from build123d import *

# Parameters (mm, degrees)
SKETCH1_W           = 13.2
SKETCH1_H           = 12.7
BOSS_EXTRUDE1_DEPTH = 9.5
SKETCH2_R           = 3
BOSS_EXTRUDE2_DEPTH = 8.8
SKETCH4_R           = 2.5
CUT_EXTRUDE1_DEPTH  = 2
SKETCH5_R           = 1.5
BOSS_EXTRUDE3_DEPTH = 13
REVOLVE2_ANGLE      = 180
FILLET1_R           = 1
SKETCH6_W           = 0.8
SKETCH6_H           = 2
BOSS_EXTRUDE4_DEPTH = 4
SKETCH7_W           = 1
SKETCH7_H           = 2
CUT_EXTRUDE2_DEPTH  = 33.182332109
FILLET2_R           = 0.5


with BuildPart() as part:
    # Sketch1 → Boss-Extrude1 (new body)
    with BuildSketch(Plane(origin=(0, 0, 0), x_dir=(1, 0, 0), z_dir=(0, 1, 0))):
        Rectangle(SKETCH1_W, SKETCH1_H)
    extrude(amount=BOSS_EXTRUDE1_DEPTH)

    # Sketch2 → Boss-Extrude2 (add)
    with BuildSketch(Plane(origin=(0, 9.5, 0), x_dir=(1, 0, 0), z_dir=(0, 1, 0))):
        with Locations(Location((0, 0, 0), (0, 0, 270))):
            Circle(SKETCH2_R)
    extrude(amount=BOSS_EXTRUDE2_DEPTH)

    # Sketch4 → Cut-Extrude1 (cut)
    with BuildSketch(Plane(origin=(0, 18.3, 0), x_dir=(1, 0, 0), z_dir=(0, 1, 0))):
        with Locations(Location((0, 0, 0), (0, 0, 270))):
            Circle(SKETCH4_R)
    extrude(amount=-CUT_EXTRUDE1_DEPTH, mode=Mode.SUBTRACT)

    # Sketch5 → Boss-Extrude3 (add)
    with BuildSketch(Plane(origin=(0, 16.3, 0), x_dir=(1, 0, 0), z_dir=(0, 1, 0))):
        with Locations(Location((0, 0, 0), (0, 0, 90))):
            Circle(SKETCH5_R)
    extrude(amount=BOSS_EXTRUDE3_DEPTH)

    # Sketch3 → Revolve2 (revolve)
    with BuildSketch(Plane(origin=(0, 16.3, 0), x_dir=(1, 0, 0), z_dir=(0, 1, 0))):
        with BuildLine():
            Line((0, -2.5), (0, 2.5))
            ThreePointArc((0, 2.5), (-2.5, 0), (0, -2.5))
        make_face()
    revolve(axis=Axis((0, 16.3, 3), (0, 0, -1)), revolution_arc=REVOLVE2_ANGLE)

    # Fillet1
    fillet1_edges = [part.edges().sort_by_distance(p)[0] for p in [
        (0, 29.3, 1.5),
    ]]
    fillet(fillet1_edges, radius=FILLET1_R)

    # Sketch6 → Boss-Extrude4 (add)
    with BuildSketch(Plane.XZ):
        with Locations((-4.7, 2.4)):
            Rectangle(SKETCH6_W, SKETCH6_H)
        with Locations((-4.7, -2.4)):
            Rectangle(SKETCH6_W, SKETCH6_H)
        with Locations((0, -2.4)):
            Rectangle(SKETCH6_W, SKETCH6_H)
        with Locations((0, 2.4)):
            Rectangle(SKETCH6_W, SKETCH6_H)
        with Locations((4.7, 2.4)):
            Rectangle(SKETCH6_W, SKETCH6_H)
        with Locations((4.7, -2.4)):
            Rectangle(SKETCH6_W, SKETCH6_H)
    extrude(amount=BOSS_EXTRUDE4_DEPTH)

    # Sketch7 → Cut-Extrude2 (cut, through all)
    with BuildSketch(Plane.ZY.offset(5.1)):
        with Locations((-2.4, -2.5)):
            Rectangle(SKETCH7_W, SKETCH7_H)
        with Locations((2.4, -2.5)):
            Rectangle(SKETCH7_W, SKETCH7_H)
    extrude(amount=-CUT_EXTRUDE2_DEPTH, mode=Mode.SUBTRACT)

    # Fillet2
    fillet2_edges = [part.edges().sort_by_distance(p)[0] for p in [
        (4.7, -3.5, 2.9),
        (4.7, -3.5, 1.9),
        (4.7, -3.5, -1.9),
        (4.7, -3.5, -2.9),
        (4.7, -1.5, -1.9),
        (4.7, -1.5, 2.9),
        (4.7, -1.5, 1.9),
        (4.7, -1.5, -2.9),
        (0, -1.5, 1.9),
        (0, -1.5, 2.9),
        (0, -3.5, 2.9),
        (0, -3.5, 1.9),
        (0, -3.5, -1.9),
        (0, -3.5, -2.9),
        (0, -1.5, -2.9),
        (0, -1.5, -1.9),
        (-4.7, -3.5, 2.9),
        (-4.7, -1.5, 2.9),
        (-4.7, -3.5, 1.9),
        (-4.7, -1.5, 1.9),
        (-4.7, -1.5, -1.9),
        (-4.7, -1.5, -2.9),
        (-4.7, -3.5, -1.9),
        (-4.7, -3.5, -2.9),
        (0, -4, -1.4),
        (0, -4, -3.4),
        (4.7, -4, -1.4),
        (4.7, -4, -3.4),
        (4.7, -4, 1.4),
        (4.7, -4, 3.4),
        (0, -4, 3.4),
        (0, -4, 1.4),
        (-4.7, -4, 3.4),
        (-4.7, -4, 1.4),
        (-4.7, -4, -1.4),
        (-4.7, -4, -3.4),
    ]]
    fillet(fillet2_edges, radius=FILLET2_R - 0.0001)  # a hair under: the kernel refuses the full size


solid = part.part
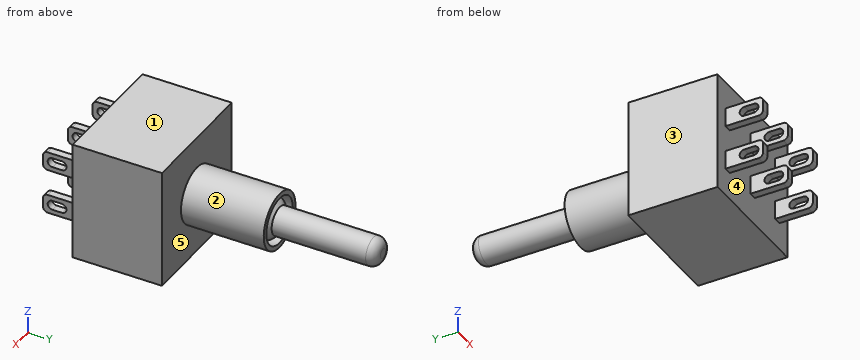
Geometry check sheet. Reference: the model listing, model coordinates, mm. Face numbers are marked on the shaded views. A direction names the side the tool comes from. Round coordinates to 2 decimals unless told otherwise and drop trailing zeros. Order: outer loops, then holes, each group sorted by start corner. A loop starts at its lowest first (then second) coordinate and runs counter-clockwise, first axis right, second up. Notation, with made-up numbers: M 0,9.25 L 7,9.25 A28 cw 7,39.25 Z; hole C 66.5,40 d5. An arc over 180 degrees is marked long. Answer in a Markdown table with one row per item.
(1) Scan lines: probe 1 along X at (y, z) = (17.25, 0); probe 2 along Z at (x, y) = (-5, -0.5); probe 3 along Y at (x, z) = (-5.5, -5). Record each from-to range of solid material in increasing order. Write a range as from..to.
Responses:
| item | result |
|---|---|
| probe 1 | x = -3..-2.5, -2.31..2.31, 2.5..3 |
| probe 2 | z = -3.4..-1.4, 1.4..3.4 |
| probe 3 | y = 0..9.5 |
(2) Go/stop test with flat-tipped pins: P1, Ø0.6, axis at y = -1.5, z = -2.5, coming from the -X side; P2, Ø0.6, axis at x = -5, y = -2.5, coming from the -Z side; P3, Ø3, axis at x = 2, z = 0, coming from the -Y side. Record where each tip stops, or that it passes through.
Responses:
| item | result |
|---|---|
| P1 | stops at x = -5.1 |
| P2 | stops at z = -3.4 |
| P3 | stops at y = 0 |
(3) Draft check along X on the marked faces 3, 4 and 5. Enter one of: released by +X, released by -X, zero draft, split by the parting line, or undercut.
Responses:
| item | result |
|---|---|
| face 3 | released by -X |
| face 4 | undercut |
| face 5 | zero draft |
(4) Sectioned sample at A-A, the plane x = 0. State how many separate pieces and enclosed holes the cut face has, and give its area (3 significant figures).
Responses:
| item | result |
|---|---|
| separate pieces | 1 |
| enclosed holes | 2 |
| area | 217 mm² |
(5) Sectioned sample at C-C, the plane x = -3.5. Record the cut outline in (y, z).
Responses:
| item | result |
|---|---|
| outline | M 0,-6.35 L 9.5,-6.35 L 9.5,6.35 L 0,6.35 Z |
(6) Tool access check on the marked faces 1 and 2. Record the directions out of +Z, -Z, +X, -X, +Y, -Y that give a thin tool (end or side, any length) a straight path to the whole face; none if there is none.
Responses:
| item | result |
|---|---|
| face 1 | +Z, +X, -X, +Y, -Y |
| face 2 | +Y |
(7) Sectioned sample at B-B, the plane z = 5.5. Record the cut outline in (x, y).
Responses:
| item | result |
|---|---|
| outline | M -6.6,0 L 6.6,0 L 6.6,9.5 L -6.6,9.5 Z |
(8) Sectioned sample at D-D, the plane y = 19. Record the cut outline in (x, z).
Responses:
| item | result |
|---|---|
| outline | C 0,0 d3 |
